Geometry check sheet. Reference: the model listing, model coordinates, mm. A direction names the side the tool comes from. Round coordinates to 2 decimals unless told otherwise and drop trailing zeros. Write each loop counter-clockwise with the first axis right and the second up, starting at its lowest first coordinate (ties: lowest second). Pieces come first, ordered by that corner, then holes.
from build123d import *

# Parameters (mm, degrees)
BOSS_EXTRUDE1_DEPTH  = 1.7
BOSS_EXTRUDE2_DEPTH  = 2
BOSS_EXTRUDE3_START  = 1.7
SKETCH3_W            = 3
SKETCH3_H            = 13.2
BOSS_EXTRUDE3_DEPTH  = 4.4
BOSS_EXTRUDE4_START  = -21
BOSS_EXTRUDE4_DEPTH  = 7.4
CUT_EXTRUDE1_START   = -21
CUT_EXTRUDE1_DEPTH   = 6
BOSS_EXTRUDE5_START  = -15
SKETCH8_W            = 6
SKETCH8_H            = 0.65
BOSS_EXTRUDE5_DEPTH  = 5
FILLET1_R            = 0.5
BOSS_EXTRUDE6_START  = 1.7
SKETCH9_W            = 5
SKETCH9_H            = 5.2
BOSS_EXTRUDE6_DEPTH  = 2
BOSS_EXTRUDE7_START  = 1.7
SKETCH10_W           = 3.35
SKETCH10_H           = 4.2
BOSS_EXTRUDE7_DEPTH  = 2
BOSS_EXTRUDE8_START  = 3.7
BOSS_EXTRUDE8_DEPTH  = 0.5
BOSS_EXTRUDE9_START  = 1.7
SKETCH12_W           = 4.5
SKETCH12_H           = 4.3
BOSS_EXTRUDE9_DEPTH  = 3.5
BOSS_EXTRUDE10_START = 1.7
SKETCH13_W           = 7.75
SKETCH13_H           = 3.3
BOSS_EXTRUDE10_DEPTH = 2.7
BOSS_EXTRUDE11_START = 1.7
SKETCH14_W           = 7
SKETCH14_H           = 7
BOSS_EXTRUDE11_DEPTH = 1
BOSS_EXTRUDE12_START = 1.7
SKETCH15_W           = 1.3
SKETCH15_H           = 2
BOSS_EXTRUDE12_DEPTH = 1
BOSS_EXTRUDE13_START = 1.7
SKETCH16_W           = 1.5
SKETCH16_H           = 2.9
BOSS_EXTRUDE13_DEPTH = 1


with BuildPart() as part:
    # Sketch1 → Boss-Extrude1 (new body)
    with BuildSketch(Plane(origin=(0, 0, 0), x_dir=(1, 0, 0), z_dir=(0, 1, 0))):
        with BuildLine():
            Line((-6.405, 21.250170418), (6.405, 21.250170418))
            Line((6.405, 21.250170418), (9.185, 15.770170418))
            ThreePointArc((9.185, 15.770170418), (0, -18.25), (-9.185, 15.770170418))
            Line((-9.185, 15.770170418), (-6.405, 21.250170418))
        make_face()
    extrude(amount=BOSS_EXTRUDE1_DEPTH)

    # Sketch2 → Boss-Extrude2 (add)
    with BuildSketch(Plane(origin=(0, 0, 0), x_dir=(1, 0, 0), z_dir=(0, 1, 0))):
        with BuildLine():
            Line((-6.75, 20.250170418), (6.75, 20.250170418))
            Line((6.75, 20.250170418), (7.794367451, 18.191489254))
            ThreePointArc((7.794367451, 18.191489254), (9.048926778, 16.291420125), (10.700777057, 14.724393497))
            ThreePointArc((10.700777057, 14.724393497), (0, -17.3), (-10.700777057, 14.724393497))
            ThreePointArc((-10.700777057, 14.724393497), (-9.048926778, 16.291420125), (-7.794367451, 18.191489254))
            Line((-7.794367451, 18.191489254), (-6.75, 20.250170418))
        make_face()
    extrude(amount=-BOSS_EXTRUDE2_DEPTH)

    # Sketch3 → Boss-Extrude3 (add)
    with BuildSketch(Plane(origin=(0, 0, 0), x_dir=(1, 0, 0), z_dir=(0, 1, 0)).offset(BOSS_EXTRUDE3_START)):
        with Locations((-13.5, 0)):
            Rectangle(SKETCH3_W, SKETCH3_H)
        with Locations((13.5, 0)):
            Rectangle(SKETCH3_W, SKETCH3_H)
    extrude(amount=BOSS_EXTRUDE3_DEPTH)

    # Sketch4 → Boss-Extrude4 (add)
    with BuildSketch(Plane.XY.offset(BOSS_EXTRUDE4_START)):
        with BuildLine():
            Line((3.5, 1.7), (-3.5, 1.7))
            ThreePointArc((-3.5, 1.7), (-4.207106781, 1.992893219), (-4.5, 2.7))
            Line((-4.5, 2.7), (-4.5, 3.7))
            ThreePointArc((-4.5, 3.7), (-4.207106781, 4.407106781), (-3.5, 4.7))
            Line((-3.5, 4.7), (3.5, 4.7))
            ThreePointArc((3.5, 4.7), (4.207106781, 4.407106781), (4.5, 3.7))
            Line((4.5, 3.7), (4.5, 2.7))
            ThreePointArc((4.5, 2.7), (4.207106781, 1.992893219), (3.5, 1.7))
        make_face()
    extrude(amount=BOSS_EXTRUDE4_DEPTH)

    # Sketch7 → Cut-Extrude1 (cut)
    with BuildSketch(Plane.XY.offset(CUT_EXTRUDE1_START)):
        with BuildLine():
            Line((4.2, 2.7), (4.2, 3.7))
            ThreePointArc((4.2, 3.7), (3.994974747, 4.194974747), (3.5, 4.4))
            Line((3.5, 4.4), (-3.5, 4.4))
            ThreePointArc((-3.5, 4.4), (-3.994974747, 4.194974747), (-4.2, 3.7))
            Line((-4.2, 3.7), (-4.2, 2.7))
            ThreePointArc((-4.2, 2.7), (-3.994974747, 2.205025253), (-3.5, 2))
            Line((-3.5, 2), (3.5, 2))
            ThreePointArc((3.5, 2), (3.994974747, 2.205025253), (4.2, 2.7))
        make_face()
    extrude(amount=CUT_EXTRUDE1_DEPTH, mode=Mode.SUBTRACT)

    # Sketch8 → Boss-Extrude5 (add)
    with BuildSketch(Plane.XY.offset(BOSS_EXTRUDE5_START)):
        with Locations((0, 3.2)):
            Rectangle(SKETCH8_W, SKETCH8_H)
    extrude(amount=-BOSS_EXTRUDE5_DEPTH)

    # Fillet1
    fillet1_edges = [part.edges().sort_by_distance(p)[0] for p in [
        (-3, 3.2, -20),
        (3, 3.2, -20),
    ]]
    fillet(fillet1_edges, radius=FILLET1_R)

    # Sketch9 → Boss-Extrude6 (add)
    with BuildSketch(Plane(origin=(0, 0, 0), x_dir=(1, 0, 0), z_dir=(0, 1, 0)).offset(BOSS_EXTRUDE6_START)):
        with Locations((6, -5.5)):
            Rectangle(SKETCH9_W, SKETCH9_H)
    extrude(amount=BOSS_EXTRUDE6_DEPTH)

    # Sketch10 → Boss-Extrude7 (add)
    with BuildSketch(Plane(origin=(0, 0, 0), x_dir=(1, 0, 0), z_dir=(0, 1, 0)).offset(BOSS_EXTRUDE7_START)):
        with Locations((10.675, -9.7)):
            Rectangle(SKETCH10_W, SKETCH10_H)
        with Locations((-10.68, -9.7)):
            Rectangle(SKETCH10_W, SKETCH10_H)
    extrude(amount=BOSS_EXTRUDE7_DEPTH)

    # Sketch11 → Boss-Extrude8 (add)
    with BuildSketch(Plane(origin=(0, 0, 0), x_dir=(1, 0, 0), z_dir=(0, 1, 0)).offset(BOSS_EXTRUDE8_START)):
        with BuildLine():
            Line((-11.78, -10.1), (-11.78, -9.3))
            ThreePointArc((-11.78, -9.3), (-10.68, -8.2), (-9.58, -9.3))
            Line((-9.58, -9.3), (-9.58, -10.1))
            ThreePointArc((-9.58, -10.1), (-10.68, -11.2), (-11.78, -10.1))
        make_face()
        with BuildLine():
            Line((9.575, -10.1), (9.575, -9.3))
            ThreePointArc((9.575, -9.3), (10.675, -8.2), (11.775, -9.3))
            Line((11.775, -9.3), (11.775, -10.1))
            ThreePointArc((11.775, -10.1), (10.675, -11.2), (9.575, -10.1))
        make_face()
    extrude(amount=BOSS_EXTRUDE8_DEPTH)

    # Sketch12 → Boss-Extrude9 (add)
    with BuildSketch(Plane(origin=(0, 0, 0), x_dir=(1, 0, 0), z_dir=(0, 1, 0)).offset(BOSS_EXTRUDE9_START)):
        with Locations((-8.852751595, 9.830469474)):
            Rectangle(SKETCH12_W, SKETCH12_H)
    extrude(amount=BOSS_EXTRUDE9_DEPTH)

    # Sketch13 → Boss-Extrude10 (add)
    with BuildSketch(Plane(origin=(0, 0, 0), x_dir=(1, 0, 0), z_dir=(0, 1, 0)).offset(BOSS_EXTRUDE10_START)):
        with Locations((-8.852751595, 10.330469474)):
            Rectangle(SKETCH13_W, SKETCH13_H)
    extrude(amount=BOSS_EXTRUDE10_DEPTH)

    # Sketch14 → Boss-Extrude11 (add)
    with BuildSketch(Plane(origin=(0, 0, 0), x_dir=(1, 0, 0), z_dir=(0, 1, 0)).offset(BOSS_EXTRUDE11_START)):
        with Locations((-3.7, -6.35)):
            Rectangle(SKETCH14_W, SKETCH14_H)
    extrude(amount=BOSS_EXTRUDE11_DEPTH)

    # Sketch15 → Boss-Extrude12 (add)
    with BuildSketch(Plane(origin=(0, 0, 0), x_dir=(1, 0, 0), z_dir=(0, 1, 0)).offset(BOSS_EXTRUDE12_START)):
        with Locations((11.85, 10.35)):
            Rectangle(SKETCH15_W, SKETCH15_H)
        with Locations((5.55, 10.35)):
            Rectangle(SKETCH15_W, SKETCH15_H)
    extrude(amount=BOSS_EXTRUDE12_DEPTH)

    # Sketch16 → Boss-Extrude13 (add)
    with BuildSketch(Plane(origin=(0, 0, 0), x_dir=(1, 0, 0), z_dir=(0, 1, 0)).offset(BOSS_EXTRUDE13_START)):
        with Locations((6, 15.8)):
            Rectangle(SKETCH16_W, SKETCH16_H)
    extrude(amount=BOSS_EXTRUDE13_DEPTH)


with BuildPart() as part_1:
    # Body-Move/Copy2: moved
    add(part.part.moved(Location((0, -15.754739533, 0))))


solid = part_1.part
1. Access from +Z, -Z, +X, -X, +Y, -Y to the whole of each face (thin tool, end or side, straight path). Record for faces 4 (the face through (-15, -12, 0)), 5 (the face through (0, -12.88, -17)), 6 (the face through (-11, -11.555, 10)), 7 (the face through (5.5, -13.6, -9.35)).
2. Section check B-B (x = 16). Record the cut outline in (y, z).
3. Release check for a two-part mould opening along Y. For faces 1 (the face through (-0.1, -13.1, -15)), 2 (the face through (-3.7, -13.6, 9.85)), 3 (the face through (0, -15.755, 18)) record: +Y half, -Y half, draft (parallel to the pull), parting line (faces both ways), or undercut.
4. Section check C-C (z = 15.5). Record the cut outline in (x, y), plus the area to 3 significant figures.
5. Scan lines: line 1 along X through (y, z) = (-12.5, -19); line 2 along X through (y, z) = (-11.75, 2.5); line 3 along X through (y, z) = (-12.5, -10). Record each from-to range of solid material in increasing order.
6. Section check A-A (z = -0.5). Record the cut outline in (x, y), plus the area to 3 significant figures.
7. Depth check by flat-ended pin: pin 1 Ø1 at (y, z) = (-11.5, -10.5) entering from -X; pin 2 Ø10 at (x, z) = (-4.5, -2.5) entering from +Y; pin 3 Ø0.9 at (x, y) = (-14, -11.5) entering from -Z. Enter the tip coordinate at first touch or a pass-through.
Results below:
1. face 4: +Z, -Z, -X, +Y
1. face 5: -Z
1. face 6: +Z, +X, -X, +Y
1. face 7: +X, +Y
2. outline: (-17.75, -8.3) - (-15.75, -8.3) - (-15.75, -8.78) - (-14.05, -8.78) - (-14.05, 8.78) - (-15.75, 8.78) - (-15.75, 7.3) - (-17.75, 7.3) - close
3. face 1: undercut
3. face 2: draft
3. face 3: -Y half
4. outline: (-9.63, -15.75) - (-7.8, -15.75) - (-7.8, -17.75) - (7.8, -17.75) - (7.8, -15.75) - (9.63, -15.75) - (9.63, -14.05) - (-9.63, -14.05) - close
4. area: 64.0 mm2
5. line 1: x = -4.5 to -4.2, -3 to 3, 4.2 to 4.5
5. line 2: x = -15 to -12, 12 to 15
5. line 3: x = -12.73 to -4.98
6. outline: (-18.24, -15.75) - (-17.8, -15.75) - (-17.8, -17.75) - (17.8, -17.75) - (17.8, -15.75) - (18.24, -15.75) - (18.24, -14.05) - (15, -14.05) - (15, -9.65) - (12, -9.65) - (12, -14.05) - (-12, -14.05) - (-12, -9.65) - (-15, -9.65) - (-15, -14.05) - (-18.24, -14.05) - close
6. area: 160 mm2
7. pin 1: stops at x = -12.73
7. pin 2: stops at y = -14.05
7. pin 3: stops at z = -6.6
